from build123d import *

# Parameters (mm, degrees)
F0_R     = 75.3277173883
F1_DEPTH = 22.606
F2_R     = 5.08
F3_R     = 5.08


with BuildPart() as f1:
    # F0 (on Top) → F1 (new body)
    with BuildSketch(Plane.XY):
        Circle(F0_R)
    extrude(amount=F1_DEPTH)

    # F2
    f2_edges = [f1.edges().sort_by_distance(p)[0] for p in [
        (-75.327717, 0, 0),
    ]]
    fillet(f2_edges, radius=F2_R)

    # F3
    f3_edges = [f1.edges().sort_by_distance(p)[0] for p in [
        (75.327717, 0, 13.843),
        (-75.327717, 0, 5.08),
        (-75.327717, 0, 22.606),
    ]]
    fillet(f3_edges, radius=F3_R)


solid = f1.part
Read the model definition and answer for the solid it produces. Units are mm, in the model's axes. Round coordinates to 2 decimals unless told otherwise and drop trailing zeros. Order: outer loops, then holes, each group sorted by start corner. A loop starts at its lowest first (then second) coordinate and runs counter-clockwise, first axis right, second up.
1) The part is cut by section A-A on z = 11.75. Write down the section's boundary in (x, y).
2) Flat-ended cylindrical pins translate along their axes: pin 1 (6 mm diameter, centred on x = -44, z = 9, fed in from -Y); pin 2 (12 mm diameter, centred on y = -27.5, z = 11, fed in from +X); pin 3 (4 mm diameter, centred on x = -30, z = 11.5, fed in from +Y). Find the tip coordinate at first contact, or state that the pin passes through.
3) Straight lines are drawn through the part: L1, parallel to X at y = -0.5, z = 15.25; L2, parallel to X at y = 66, z = 20; L3, parallel to Y at x = 21.5, z = 17.75. For each, find the intervals that lie inside material, in ascending order.
Resolved:
1. outline: circle Ø150.66 at (0, 0)
2. pin 1: stops at y = -63.19
2. pin 2: stops at x = 72.19
2. pin 3: stops at y = 69.93
3. L1: x = -75.33 to 75.33
3. L2: x = -34.95 to 34.95
3. L3: y = -72.19 to 72.19
